Could you check a few things on this drawing? It's one solid part, dimensions in mm from its lowest x, y, z. A direction names the side the tool comes from. Round coordinates to 2 decimals unless told otherwise and drop trailing zeros. Loops run counter-clockwise (first coordinate to the right, second up) from the corner with the lowest first, then second, coordinate; pieces in that order, holes last. Notation, with made-up numbers: (47.5, 74.25) -> (91.5, 74.25) arc R35 ccw to (91.5, 109.25) -> close; hole circle Ø1 at (57, 2). An arc over 180 degrees is marked (long way). Write each question's results on one line, items separated by ' | '.
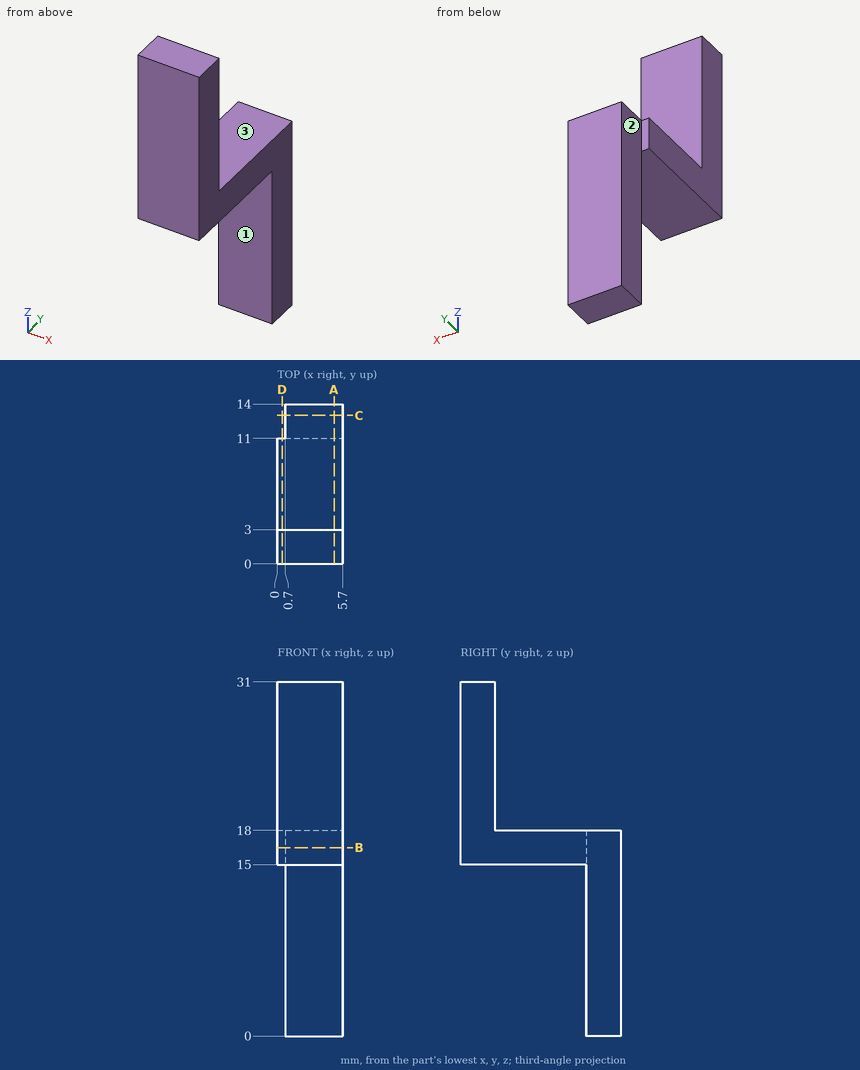
1) I want a section at A-A, the plane x = 4.95. Write out the boundary of the cut face in (y, z), plus the area to 3 significant figures.
Model answer:
outline: (0, 15) -> (11, 15) -> (11, 0) -> (14, 0) -> (14, 18) -> (3, 18) -> (3, 31) -> (0, 31) -> close | area: 126 mm2
2) I need wall thicknesses on line 1 (X direction, y = 11.25, z = 9.5); line 2 (Z direction, x = 1.2, y = 4.75); line 3 (Z direction, x = 3.65, y = 2). Which ranges of each line are inside material? Lowest first, please.
Model answer:
line 1: x = 0.7 to 5.7 | line 2: z = 15 to 18 | line 3: z = 15 to 31
3) I want a section at D-D, the plane x = 0.4. Write out the boundary of the cut face in (y, z), plus the area to 3 significant figures.
Model answer:
outline: (0, 15) -> (11, 15) -> (11, 18) -> (3, 18) -> (3, 31) -> (0, 31) -> close | area: 72.0 mm2
4) I'm going to push flat-ended pins straight in: pin 1 (1.5 mm diameter, centred on x = 1, y = 4.5, fed in from -Z); pin 2 (1 mm diameter, centred on x = 4, y = 11, fed in from +Z); pin 3 (8 mm diameter, centred on y = 8.5, z = 5, fed in from -X). Where does each tip first touch, or does it pass through?
Model answer:
pin 1: stops at z = 15 | pin 2: stops at z = 18 | pin 3: stops at x = 0.7
5) I want a section at C-C, the plane y = 13. Write out the boundary of the cut face in (x, z).
Model answer:
outline: (0.7, 0) -> (5.7, 0) -> (5.7, 18) -> (0.7, 18) -> close
6) For the marked faces 1, 2 and 3, which set-ups out of +Z, -Z, +X, -X, +Y, -Y let a thin tool reach every point of the face, with its end or its side?
Model answer:
face 1: -Z, +X, -X, -Y | face 2: +Z, -Z, -X, +Y | face 3: +Z, +X, -X, +Y
7) I want a section at B-B, the plane z = 16.5. Write out the boundary of the cut face in (x, y), plus the area to 3 significant figures.
Model answer:
outline: (0, 0) -> (5.7, 0) -> (5.7, 14) -> (0.7, 14) -> (0.7, 11) -> (0, 11) -> close | area: 77.7 mm2
